Input: part model. Units: mm. Frame: model coordinates. Face numbers are marked on the shaded views. A direction names the side the tool comes from. Give positions to 0.01 mm unless a question says otherwise; leave off trailing zeros. Loops run counter-clockwise (first coordinate to the right, second up) from the corner with the lowest first, then second, coordinate; pieces in that order, holes last. Notation, with made-up numbers: (-1, 87.5) - (5, 87.5) arc R14 cw to (5, 108.5) - close; hole circle Ø8 at (83.25, -8.75). An arc over 180 degrees is marked (long way). Answer as a JSON object with one key per item and string values. Group by question number.
(1) Mould query, pull axis X, two halves, no side actions, for the marked faces 1, 2 and 3. Classes: +X half, -X half, draft (parallel to the pull), parting line (faces both ways), or undercut.
(2) Material intervals for L1, parallel to Z at x = 38.1, y = 74.85; L2, parallel to Z at x = 150.2, y = 31.75; L3, parallel to X at y = 36.5, z = 78.5, sorted ascending.
(3) Section query B-B (y = 18.5). Return loops of the section in (x, z).
(4) Section query A-A (x = 57.15). Return loops of the section in (y, z), plus the area to 3 significant figures.
(5) Section query C-C (z = 12.7). Count the separate pieces of the cut face and the enclosed holes in it, plus the area to 3 significant figures.
(6) Section query D-D (y = 31.75). Return loops of the section in (x, z), plus the area to 3 significant figures.
(7) Pin query (flat end, axial travel): P1, Ø8, axis at y = 31.75, z = 63.5, coming from the +X side; P2, Ø5, axis at x = 33.5, z = 114, coming from the -Y side. Return the tip coordinate at first contact, or that it passes through.
(8) Access query for the marked faces 4 and 5. Directions: +Z, -Z, +X, -X, +Y, -Y. A direction counts if a zero-diameter tool reaches every point of the face in a straight line with its end or side. Return the directions, or none.
Autodesk Inventor part; units mm, degrees
ref_plane "YZ Plane" through (0, 0, 0) normal (1, 0, 0) x (0, 1, 0)
ref_plane "XZ Plane" through (0, 0, 0) normal (0, 1, 0) x (-1, 0, 0)
ref_plane "XY Plane" through (0, 0, 0) normal (0, 0, 1) x (1, 0, 0)
sketch "Sketch1" plane through (0, 0, 0) normal (0, 0, 1) x (1, 0, 0)
  line L0 (0, 0) -> (0, 66.675)
  line L1 (9.525, 76.2) -> (142.875, 76.2)
  line L2 (152.4, 66.675) -> (152.4, 0)
  line L3 (152.4, 0) -> (149.3622, 0)
  line L4 (149.3622, 0) -> (149.3622, 66.8122)
  line L5 (143.0122, 73.1622) -> (9.3878, 73.1622)
  line L6 (3.0378, 66.8122) -> (3.0378, 0)
  line L7 (3.0378, 0) -> (0, 0)
  arc A0 (9.3878, 73.1622) -> (3.0378, 66.8122) centre (9.3878, 66.8122) ccw
  arc A1 (149.3622, 66.8122) -> (143.0122, 73.1622) centre (143.0122, 66.8122) ccw
  arc A2 (9.525, 76.2) -> (0, 66.675) centre (9.525, 66.675) ccw
  arc A3 (152.4, 66.675) -> (142.875, 76.2) centre (142.875, 66.675) ccw
  point P0 (0, 76.2)
  point P1 (152.4, 76.2)
  dimension "d0" = 76.2
  dimension "d1" = 3.0378
  dimension "d2" = 3.0378
  dimension "d3" = 152.4
  dimension "d4" = 6.35
  dimension "d5" = 9.525
extrude "Extrusion1" add sketch "Sketch1" along normal blind 127
hole "Hole1" at (25.4, 76.2, 63.5) direction (0, -1, 0) diameter 9.906 end through all
pattern_linear "Rectangular Pattern1" count 2 spacing 31.75 along (1, 0, 0) of "Hole1"
hole "Hole2" at (0, 31.75, 63.5) direction (1, 0, 0) diameter 9.906 end through all
hole "Hole3" at (38.1, 73.1622, 12.7) direction (0, 1, 0) diameter 6.731 depth 25.4 tip angle 118
pattern_linear "Rectangular Pattern2" count 2 spacing 76.2 along (1, 0, 0) count 2 spacing 101.6 along (0, 0, 1) of "Hole3"
equation "\"d2\" = d1"
properties part number "GE-12025" material "Steel"
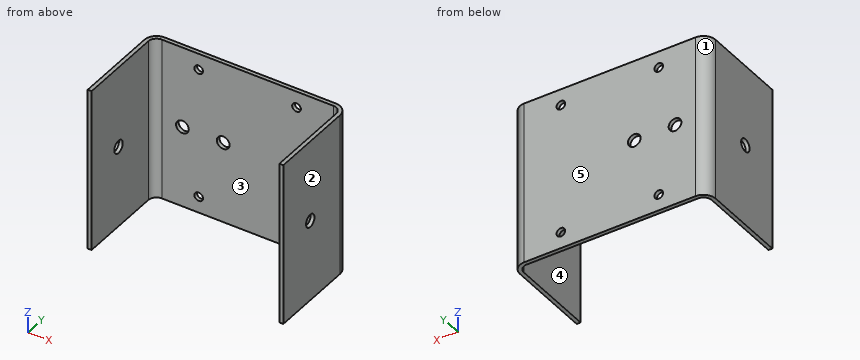
Recorded:
{
 "1": {"face 1": "-X half", "face 2": "+X half", "face 3": "undercut"},
 "2": {"L1": "z = 0 to 9.33, 16.07 to 110.93, 117.67 to 127", "L2": "z = 0 to 58.55, 68.45 to 127", "L3": "x = 0 to 3.04, 149.36 to 152.4"},
 "3": {"outline": "(0, 0) - (3.04, 0) - (3.04, 127) - (0, 127) - close; (149.36, 0) - (152.4, 0) - (152.4, 127) - (149.36, 127) - close"},
 "4": {"outline": "(73.16, 0) - (76.2, 0) - (76.2, 58.55) - (73.16, 58.55) - close; (73.16, 68.45) - (76.2, 68.45) - (76.2, 127) - (73.16, 127) - close", "area": "356 mm^2"},
 "5": {"separate pieces": "3", "enclosed holes": "0", "area": "845 mm^2"},
 "6": {"outline": "(0, 0) - (3.04, 0) - (3.04, 58.55) - (0, 58.55) - close; (0, 68.45) - (3.04, 68.45) - (3.04, 127) - (0, 127) - close; (149.36, 0) - (152.4, 0) - (152.4, 58.55) - (149.36, 58.55) - close; (149.36, 68.45) - (152.4, 68.45) - (152.4, 127) - (149.36, 127) - close", "area": "711 mm^2"},
 "7": {"P1": "passes through", "P2": "stops at y = 73.16"},
 "8": {"face 4": "+Z, -Z, -Y", "face 5": "+Z, -Z, +X, -X, +Y"}
}
